Autodesk Inventor part; units mm, degrees
ref_plane "Work Plane1" through (0, -100, 0) normal (0, 1, 0) x (-1, 0, 0)
ref_plane "YZ Plane" through (0, 0, 0) normal (1, 0, 0) x (0, 1, 0)
ref_plane "XY Plane" through (0, 0, 0) normal (0, 0, 1) x (1, 0, 0)
sketch "Sketch1" plane through (0, 0, 0) normal (0, 0, 1) x (1, 0, 0)
  line L0 (0, -110.6871) -> (0, 217.0976)
  line L1 (144, 0) -> (144, -18)
  arc A0 (121.1146, -57.8857) -> (144, -18) centre (97.8, -18) ccw
  arc A1 (0, -90.6871) -> (121.1146, -57.8857) centre (0, 149.3129) ccw
  line L2 (144, 0) -> (190, 0)
  line L3 (144, -18) -> (97.8, -18) construction
  line L4 (121.1146, -57.8857) -> (97.8, -18) construction
  line L5 (0, -90.6871) -> (0, -110.6871) construction
  line L6 (0, -110.6871) -> (190, -110.6871)
  line L7 (190, -110.6871) -> (190, 0)
  line L8 (0, -90.6871) -> (0, -110.6871)
  line L9 (144, 0) -> (190, 0)
  point P0 (0, 0)
  dimension "d0" = 288
  dimension "d19" = 380
  dimension "d20" = 20
  dimension "d22" = 18
  dimension "d23" = 46.2
  dimension "d24" = 240
  dimension "d26" = 46
revolve "Revolution1" add sketch "Sketch1" angle 360 about axis through (0, -110.6871, 0) along (0, 1, 0)
ref_plane "Work Plane1" through (0, -100, 0) normal (0, 1, 0) x (-1, 0, 0)
sketch "Sketch2" plane through (0, -110.6871, 0) normal (0, -1, 0) x (1, 0, 0)
  circle A0 centre (0, 0) radius 190 construction
  point P0 (0, 0)
  point P1 (0, -175)
  point P2 (0, 0)
  dimension "d8" = 175
hole "Hole1" at (0, -110.6871, -175) direction (0, 1, 0) diameter 8.376 end through all
pattern_circular "Circular Pattern1" count 18 over 360 about axis through (0, -9, 0) along (0, 1, 0) of "Hole1"
properties part number "Korbbogenboden"
Source: CAD feature listing. Evaluate the final solid. Frame: model axes, mm. Give positions to 0.01 mm unless a question says otherwise; leave off trailing zeros. Write each loop counter-clockwise with the first axis right and the second up, starting at its lowest first coordinate (ties: lowest second). Pieces come first, ordered by that corner, then holes. Notation, with made-up numbers: (25.25, 26.5) - (34.25, 26.5) arc R19 ccw to (34.25, 56.5) - close; hole circle Ø11 at (5.25, -21). An arc over 180 degrees is marked (long way). Write item = value, one per line. Start each with the question number.
Q1. Cut plane B-B, the plane z = 152. Return loops of the section in (x, y), then the cut area to 3 significant figures.
Q2. Pin query (flat end, axial travel): pin 1 Ø6.5 at (x, z) = (59.85, -164.45) entering from +Y; pin 2 Ø9.5 at (x, z) = (-59.85, 164.45) entering from +Y; pin 3 Ø10 at (x, y) = (80, -29) entering from +Z; pin 4 Ø8 at (y, z) = (-70, 112) entering from +X. Return the tip coordinate at first contact, or that it passes through.
Q3. Material intervals for probe 1 along Y at (x, z) = (84, 92); probe 2 along Z at (x, y) = (-152.5, -27); probe 3 along Z at (x, y) = (82, -24.5), sorted ascending.
Q4. Cut plane D-D, the plane x = -162. Return loops of the section in (y, z).
Q5. Draft query along Z for faces 1 (the cylindrical face through (175.9, -54.6, 32.6)), 2 (the flat face through (27, 0, -142)), 3 (the cylindrical face through (-41.19, -54.57, 185.48)). Return one class per face: +Z half, -Z half, draft (parallel to the pull), parting line (faces both ways), or undercut.
Computed values:
q1.outline = (-114, -110.69) - (114, -110.69) - (114, 0) - (-114, 0) - close
q1.area = 25,200 mm²
q2.pin_1 = through
q2.pin_2 = 0
q2.pin_3 = 174.57
q2.pin_4 = 156.32
q3.probe_1 = -110.69 to -55.65
q3.probe_2 = -113.33 to -91.58, -83.42 to 83.42, 91.58 to 113.33
q3.probe_3 = -171.39 to -117.81, 117.81 to 171.39
q4.outline = (-110.69, -99.28) - (0, -99.28) - (0, 99.28) - (-110.69, 99.28) - close
q5.face_1 = undercut
q5.face_2 = draft
q5.face_3 = parting line
